Autodesk Inventor part; units mm, degrees
ref_plane "YZ Plane" through (0, 0, 0) normal (1, 0, 0) x (0, 1, 0)
ref_plane "XZ Plane" through (0, 0, 0) normal (0, 1, 0) x (-1, 0, 0)
ref_plane "XY Plane" through (0, 0, 0) normal (0, 0, 1) x (1, 0, 0)
sketch "Sketch1" plane through (0, 0, 0) normal (1, 0, 0) x (0, 1, 0)
  circle A0 centre (0, 0) radius 7.5985
  dimension "d0" = 15.197
extrude "Extrusion1" add sketch "Sketch1" along normal blind 1.28
sketch "Sketch2" plane through (1.28, 0, 0) normal (1, 0, 0) x (0, 0, -1)
  line L0 (3.6604, 6.34) -> (7.3208, 0)
  line L1 (7.3208, 0) -> (3.6604, -6.34)
  line L2 (3.6604, -6.34) -> (-3.6604, -6.34)
  line L3 (-3.6604, -6.34) -> (-7.3208, 0)
  line L4 (-7.3208, 0) -> (-3.6604, 6.34)
  line L5 (-3.6604, 6.34) -> (3.6604, 6.34)
  point P0 (0, 0)
  point P1 (0, 6.34)
  point P2 (0, 0)
extrude "Extrusion2" add sketch "Sketch2" along normal blind 7.5
sketch "Sketch3" plane through (8.78, 0, 0) normal (1, 0, 0) x (0, 0, -1)
  circle A0 centre (0, 0) radius 5.927
  dimension "d5" = 11.854
extrude "Extrusion3" add sketch "Sketch3" along normal blind 1.22
sketch "Sketch4" plane through (10, 0, 0) normal (1, 0, 0) x (0, 0, -1)
  circle A0 centre (0, 0) radius 6.34
  line L0 (3.6604, 6.34) -> (-3.6604, 6.34)
extrude "Extrusion4" add sketch "Sketch4" along normal blind 1.5
fillet "Fillet1" radius 0.75 5 edges at (5.03, 0, -7.3208) (5.03, -6.34, -3.6604) (5.03, 0, 7.3208) (5.03, 6.34, -3.6604) (5.03, 6.34, 3.6604)
fillet "Fillet2" radius 0.75 1 edges at (5.03, -6.34, 3.6604)
sketch "Sketch5" plane through (0, 0, 0) normal (-1, 0, 0) x (0, 0, 1)
  point P0 (0, 0)
sketch "Sketch6" plane through (1.28, 6.34, 3.2274) normal (0, 1, 0) x (1, 0, 0)
  circle A0 centre (3.75, 3.2274) radius 1.3525
  point P0 (-1.28, 3.2274)
  dimension "d12" = 2.705
extrude "Extrusion5" cut sketch "Sketch6" against normal blind 6.5
sketch "Sketch7" plane through (0, 0, 0) normal (-1, 0, 0) x (0, 0, 1)
  circle A0 centre (0, 0) radius 3.2
  dimension "d15" = 6.4
sketch "Sketch8" plane through (5.03, -0.16, 0) normal (0, 1, 0) x (1, 0, 0)
  point P0 (-5.03, 0)
extrude "Extrusion6" cut sketch "Sketch7" against normal blind 11.75
sketch "Sketch9" plane through (0, 0, 0) normal (-1, 0, 0) x (0, 0, 1)
  circle A0 centre (0, 0) radius 3.2
  circle A1 centre (0, 0) radius 4.2
  dimension "d18" = 8.4
extrude "Extrusion7" add sketch "Sketch9" along normal blind 5
fillet "Fillet3" radius 2 1 edges at (0, 0, -4.2)
properties part number "_3DPrint"
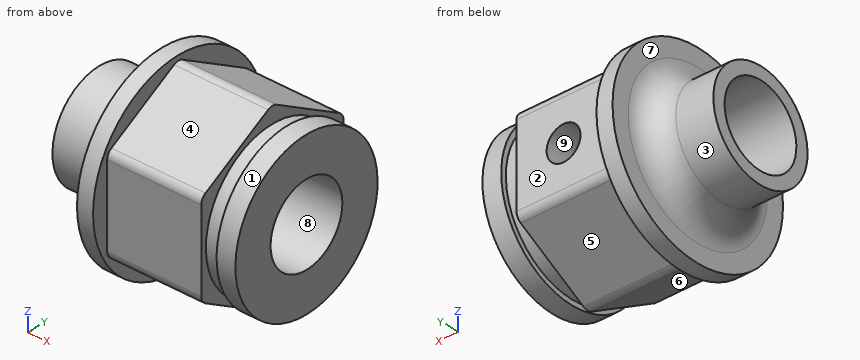
Here's how the part is built. I have some questions about the finished solid (model axes, mm). Face numbers are marked on the shaded views. A direction names the side the tool comes from. Round coordinates to 2 decimals unless told otherwise and drop trailing zeros. Write each loop counter-clockwise with the first axis right and the second up, starting at its lowest first coordinate (ties: lowest second). Pieces come first, ordered by that corner, then holes.
1. I need wall thicknesses on L1, parallel to Y at x = 7.5, z = 0; L2, parallel to X at y = 3.85, z = 0; L3, parallel to X at y = -3.75, z = 5.75. Which ranges of each line are inside material? Lowest first, please.
2. Suppose I cut it at C-C (x = 1.75). List the corners of the cut face in (y, z) for me (3 decimals).
3. If we mould it in two halves opening along Z, with no side actions, what happens to the marked faces 6, 7, 8 and 9? For each: released by +Z, released by -Z, zero draft, split by the parting line, or undercut.
4. Suppose I cut it at B-B (z = 0). State how many separate pieces and enclosed holes the cut face has, and give its area (3 significant figures).
5. Suppose I cut it at A-A (y = 0). List the corners of the cut face in (x, z) for me.
6. Will these pins go through, and if not, where does the flat tip stop? pin 1 Ø3 at (x, z) = (9.5, -5) entering from +Y; pin 2 Ø7 at (x, z) = (6, 1) entering from +Y; pin 3 Ø2 at (x, y) = (5.5, 4) entering from -Z; pin 4 Ø4 at (y, z) = (0, 0) entering from +X.
7. Suppose I cut it at D-D (x = 5.5). List the corners of the cut face in (y, z) for me (3 decimals).
8. For the marked faces 1, 2, 3, 4 and 5, which set-ups out of +Z, -Z, +X, -X, +Y, -Y let a thin tool reach every point of the face, with its end or its side?
Answer sheet:
1. L1: y = -6.34 to -3.2, 3.2 to 6.34
1. L2: x = -5 to 3.68, 6.38 to 11.5
1. L3: x = 0 to 1.28
2. outline: (-6.34, -3.227) arc R0.75 ccw to (-5.965, -3.877) - (-0.375, -7.104) arc R0.75 ccw to (0.375, -7.104) - (5.965, -3.877) arc R0.75 ccw to (6.34, -3.227) - (6.34, 3.227) arc R0.75 ccw to (5.965, 3.877) - (0.375, 7.104) arc R0.75 ccw to (-0.375, 7.104) - (-5.965, 3.877) arc R0.75 ccw to (-6.34, 3.227) - close; hole circle Ø6.4 at (0, 0)
3. face 6: released by -Z
3. face 7: zero draft
3. face 8: undercut
3. face 9: undercut
4. separate pieces: 3
4. enclosed holes: 0
4. area: 77.7 mm2
5. outline: (-5, -4.2) - (-2, -4.2) arc R2 cw to (0, -6.2) - (0, -7.6) - (1.28, -7.6) - (1.28, -7.2) - (8.78, -7.2) - (8.78, -5.93) - (10, -5.93) - (10, -6.34) - (11.5, -6.34) - (11.5, -3.2) - (-5, -3.2) - close; (-5, 3.2) - (11.5, 3.2) - (11.5, 6.34) - (10, 6.34) - (10, 5.93) - (8.78, 5.93) - (8.78, 7.2) - (1.28, 7.2) - (1.28, 7.6) - (0, 7.6) - (0, 6.2) arc R2 cw to (-2, 4.2) - (-5, 4.2) - close
6. pin 1: stops at y = 6.18
6. pin 2: stops at y = 6.34
6. pin 3: stops at z = -5.59
6. pin 4: passes through
7. outline: (-6.34, -3.227) arc R0.75 ccw to (-5.965, -3.877) - (-0.375, -7.104) arc R0.75 ccw to (0.375, -7.104) - (5.965, -3.877) arc R0.75 ccw to (6.34, -3.227) - (6.34, -1.268) - (2.938, -1.268) arc R3.2 cw (long way) to (2.938, 1.268) - (6.34, 1.268) - (6.34, 3.227) arc R0.75 ccw to (5.965, 3.877) - (0.375, 7.104) arc R0.75 ccw to (-0.375, 7.104) - (-5.965, 3.877) arc R0.75 ccw to (-6.34, 3.227) - close
8. face 1: +X
8. face 2: +Z, -Z, +X, +Y
8. face 3: -X
8. face 4: +Z, +X, -Y
8. face 5: -Z, +X, +Y
